```python
from build123d import *

# Parameters (mm, degrees)
SKETCH1_R           = 10
BOSS_EXTRUDE1_DEPTH = 0.5
SKETCH4_R           = 14
BOSS_EXTRUDE3_DEPTH = 2
SKETCH5_R           = 10
BOSS_EXTRUDE4_DEPTH = 0.5
SKETCH6_R           = 7.5
BOSS_EXTRUDE6_DEPTH = 5
SKETCH7_R           = 1.55
CUT_EXTRUDE1_DEPTH  = 22.354156504


with BuildPart() as part:
    # Sketch1 → Boss-Extrude1 (new body)
    with BuildSketch(Plane.XY):
        Circle(SKETCH1_R)
    extrude(amount=BOSS_EXTRUDE1_DEPTH)

    # Sketch4 → Boss-Extrude3 (add)
    with BuildSketch(Plane.XY.offset(0.5)):
        Circle(SKETCH4_R)
    extrude(amount=BOSS_EXTRUDE3_DEPTH)

    # Sketch5 → Boss-Extrude4 (add)
    with BuildSketch(Plane.XY.offset(2.5)):
        Circle(SKETCH5_R)
    extrude(amount=BOSS_EXTRUDE4_DEPTH)

    # Sketch6 → Boss-Extrude6 (add)
    with BuildSketch(Plane.XY.offset(3)):
        with Locations((1.5, 0)):
            Circle(SKETCH6_R)
    extrude(amount=BOSS_EXTRUDE6_DEPTH)

    # Sketch7 → Cut-Extrude1 (cut, through all)
    with BuildSketch(Plane.XY.offset(8)):
        with Locations((0, 3)):
            Circle(SKETCH7_R)
        with Locations(Location((0, -3, 0), (0, 0, 180))):
            Circle(SKETCH7_R)
    extrude(amount=-CUT_EXTRUDE1_DEPTH, mode=Mode.SUBTRACT)


solid = part.part
```
CAD build for the part. Positions are in the model's coordinates, mm. A direction names the side the tool comes from. Coordinates: 2 decimals unless noted, no trailing zeros. Write each loop counter-clockwise with the first axis right and the second up, starting at its lowest first coordinate (ties: lowest second). Pieces come first, ordered by that corner, then holes. Notation, with made-up numbers: (59, 17) -> (106, 17) arc R12 ccw to (106, 27) -> close; hole circle Ø4 at (68.25, 55). An arc over 180 degrees is marked (long way). Return JSON: item names as keys, results as strings. Group by question number.
Q1. Pull direction Y, two halves, no side cores. Call faces 1 (the face through (0, 0, 0)), 2 (the face through (0.336, -1.487, 4.056)), 3 (the face through (-2.17, -9.76, 2.75)): released by +Y, released by -Y, zero draft, split by the parting line, or undercut.
Q2. Flat gauge pins, fed straight in: pin 1 (3 mm diameter, centred on y = -2, z = 5.5, fed in from +X); pin 2 (3 mm diameter, centred on x = 0, y = 3, fed in from -Z); pin 3 (6 mm diameter, centred on x = -5, y = 7.5, fed in from +Z); pin 4 (1.5 mm diameter, centred on x = 5.5, z = 6, fed in from +Y). Where does each tip first touch, or does it go through?
Q3. Cut at B-B, the plane x = 0. Give the cut face in (y, z), then the cut area to 3 significant figures.
Q4. Drill centre lines: line 1 (Y direction, x = 0, z = 5); line 2 (Z direction, x = -11.5, y = -5.25); line 3 (X direction, y = -3, z = 5.5). Where is each one in solid material? Low to high.
Q5. Cut at C-C, the plane z = 1.5. Give the cut face in (x, y).
Q6. Cut at D-D, the plane y = 3. Give the cut face in (x, z), then the cut area to 3 significant figures.
Q7. Cut at A-A, the plane y = 0. Give the cut face in (x, z), then the cut area to 3 significant figures.
Q8. Which spindle directions (+Z, -Z, +X, -X, +Y, -Y) get a long thin tool onto all of the face, cutting with end or side? Do faces 4 (the face through (-3, 10, 2.5)), 5 (the face through (-3, 10, 0.5)), 6 (the face through (12.932, -5.362, 1.486)). Say none if no direction does.
Returned:
{
 "1": {"face 1": "zero draft", "face 2": "undercut", "face 3": "split by the parting line"},
 "2": {"pin 1": "stops at x = 8.98", "pin 2": "passes through", "pin 3": "stops at z = 8", "pin 4": "stops at y = 6.76"},
 "3": {"outline": "(-14, 0.5) -> (-10, 0.5) -> (-10, 0) -> (-4.55, 0) -> (-4.55, 8) -> (-7.35, 8) -> (-7.35, 3) -> (-10, 3) -> (-10, 2.5) -> (-14, 2.5) -> close; (-1.45, 0) -> (1.45, 0) -> (1.45, 8) -> (-1.45, 8) -> close; (4.55, 0) -> (10, 0) -> (10, 0.5) -> (14, 0.5) -> (14, 2.5) -> (10, 2.5) -> (10, 3) -> (7.35, 3) -> (7.35, 8) -> (4.55, 8) -> close", "area": "99.9 mm2"},
 "4": {"line 1": "y = -7.35 to -4.55, -1.45 to 1.45, 4.55 to 7.35", "line 2": "z = 0.5 to 2.5", "line 3": "x = -5.37 to -1.55, 1.55 to 8.37"},
 "5": {"outline": "circle Ø28 at (0, 0); hole circle Ø3.1 at (0, -3); hole circle Ø3.1 at (0, 3)"},
 "6": {"outline": "(-13.67, 0.5) -> (-9.54, 0.5) -> (-9.54, 0) -> (-1.55, 0) -> (-1.55, 8) -> (-5.37, 8) -> (-5.37, 3) -> (-9.54, 3) -> (-9.54, 2.5) -> (-13.67, 2.5) -> close; (1.55, 0) -> (9.54, 0) -> (9.54, 0.5) -> (13.67, 0.5) -> (13.67, 2.5) -> (9.54, 2.5) -> (9.54, 3) -> (8.37, 3) -> (8.37, 8) -> (1.55, 8) -> close", "area": "118 mm2"},
 "7": {"outline": "(-14, 0.5) -> (-10, 0.5) -> (-10, 0) -> (10, 0) -> (10, 0.5) -> (14, 0.5) -> (14, 2.5) -> (10, 2.5) -> (10, 3) -> (9, 3) -> (9, 8) -> (-6, 8) -> (-6, 3) -> (-10, 3) -> (-10, 2.5) -> (-14, 2.5) -> close", "area": "151 mm2"},
 "8": {"face 4": "+Z", "face 5": "-Z", "face 6": "+Z, -Z"}
}
